Autodesk Inventor part; units mm, degrees
ref_plane "YZ Plane" through (0, 0, 0) normal (1, 0, 0) x (0, 1, 0)
ref_plane "XZ Plane" through (0, 0, 0) normal (0, 1, 0) x (-1, 0, 0)
ref_plane "XY Plane" through (0, 0, 0) normal (0, 0, 1) x (1, 0, 0)
sketch "Sketch1" plane through (0, 0, 0) normal (0, 0, 1) x (1, 0, 0)
  line L0 (0, 0) -> (50, 0) construction
  line L1 (0, -5) -> (50, -5)
  line L2 (50, 5) -> (0, 5)
  arc A0 (0, 5) -> (0, -5) centre (0, 0) ccw
  arc A1 (50, -5) -> (50, 5) centre (50, 0) ccw
  line L3 (0, 0) -> (50, 0) construction
  circle A2 centre (0, 0) radius 1.5
  circle A3 centre (50, 0) radius 1.5
  circle A4 centre (30, 0) radius 1.5
  point P0 (25, 0)
  dimension "d0" = 50
  dimension "d1" = 0
  dimension "d2" = 10
  dimension "d3" = 3
  dimension "d4" = 3
  dimension "d5" = 3
  dimension "d6" = 20
extrude "Extrusion1" add sketch "Sketch1" along normal blind 5
sketch "Sketch2" plane through (0, 0, 5) normal (0, 0, 1) x (1, 0, 0)
  arc A0 (50, -5) -> (50, 5) centre (50, 0) ccw
  line L0 (50, 5) -> (0, 5)
  arc A1 (0, 5) -> (0, -5) centre (0, 0) ccw
  line L1 (0, -5) -> (50, -5)
  circle A2 centre (30, 0) radius 1.5
  circle A3 centre (50, 0) radius 1.5
  circle A4 centre (0, 0) radius 1.5
properties part number "Arm3_3D" material "Aluminum 6061, Welded"
Check sheet for the modelled part. Datum: model origin and axes. Units: mm. Round coordinates to 2 decimals unless told otherwise and drop trailing zeros. Write each loop counter-clockwise with the first axis right and the second up, starting at its lowest first coordinate (ties: lowest second). Pieces come first, ordered by that corner, then holes. Notation, with made-up numbers: (25.25, 79) - (74.25, 79) arc R21 ccw to (74.25, 94) - close; hole circle Ø9 at (82.5, 86.5). An arc over 180 degrees is marked (long way). Return JSON: item names as keys, results as strings.
Q1. Cross-section at B-B (z = 4.25). Record the boundary of the cut face in (x, y).
Returned:
{"outline": "(0, -5) - (50, -5) arc R5 ccw to (50, 5) - (0, 5) arc R5 ccw to start; hole circle Ø3 at (0, 0); hole circle Ø3 at (30, 0); hole circle Ø3 at (50, 0)"}
Q2. Scan lines: L1, parallel to Y at x = 30, z = 3.25; L2, parallel to X at y = -1.25, z = 0.6; L3, parallel to X at y = 0.25, z = 2.3. Record each from-to range of solid material in increasing order. Write a range as from..to.
Returned:
{"L1": "y = -5..-1.5, 1.5..5", "L2": "x = -4.84..-0.83, 0.83..29.17, 30.83..49.17, 50.83..54.84", "L3": "x = -4.99..-1.48, 1.48..28.52, 31.48..48.52, 51.48..54.99"}
Q3. Cross-section at D-D (y = 4). Record the boundary of the cut face in (x, z).
Returned:
{"outline": "(-3, 0) - (53, 0) - (53, 5) - (-3, 5) - close"}
Q4. Draft check along Y on faces 1 (the flat face through (25, 5, 2)), 2 (the flat face through (25, 0, 5)), 3 (the cylindrical face through (-1.5, -0.07, 2.46)), 4 (the cylindrical face through (28.5, -0.07, 2.46)). Enter one of: released by +Y, released by -Y, zero draft, split by the parting line, or undercut.
Returned:
{"face 1": "released by +Y", "face 2": "zero draft", "face 3": "undercut", "face 4": "undercut"}
Q5. Depth check by flat-ended pin: P1, Ø3, axis at y = -2.5, z = 0.5, coming from the +X side; P2, Ø2.5, axis at x = 0, y = 0, coming from the +Z side. Enter the tip coordinate at first touch or a pass-through.
Returned:
{"P1": "stops at x = 54.9", "P2": "passes through"}
Q6. Cross-section at C-C (x = 30). Record the boundary of the cut face in (y, z).
Returned:
{"outline": "(-5, 0) - (-1.5, 0) - (-1.5, 5) - (-5, 5) - close; (1.5, 0) - (5, 0) - (5, 5) - (1.5, 5) - close"}
Q7. Cross-section at A-A (y = 0). Record the boundary of the cut face in (x, z).
Returned:
{"outline": "(-5, 0) - (-1.5, 0) - (-1.5, 5) - (-5, 5) - close; (1.5, 0) - (28.5, 0) - (28.5, 5) - (1.5, 5) - close; (31.5, 0) - (48.5, 0) - (48.5, 5) - (31.5, 5) - close; (51.5, 0) - (55, 0) - (55, 5) - (51.5, 5) - close"}
